Check sheet for the modelled part. Datum: model origin and axes. Units: mm. Face numbers are marked on the shaded views. Give positions to 0.01 mm unless a question says otherwise; leave off trailing zeros. Loops run counter-clockwise (first coordinate to the right, second up) from the corner with the lowest first, then second, coordinate; pieces in that order, holes last. Notation, with made-up numbers: (11.5, 20.5) -> (46.5, 20.5) arc R23 ccw to (46.5, 57.5) -> close; hole circle Ø3 at (27, 9.25). An arc over 180 degrees is marked (long way). Answer as CSV lines item,"result". Start each with the question number.
(1) Gauge pin test, flat ends, axial feed: pin 1 Ø5 at (x, z) = (120, 10.5) entering from -Y; pin 2 Ø0.6 at (y, z) = (3.5, 15.5) entering from -X; pin 3 Ø1.5 at (y, z) = (1.5, 9.5) entering from +X. Record the tip position at first contact, or that the pin passes through.
(2) Release check for a two-part mould opening along Z. For the marked faces 1 and 2 record: pulls with the +Z half, pulls with the -Z half, needs draft (parallel to the pull), parting line crosses it, or undercut.
(3) Section check A-A on x = 51.5. Enter the section's corners in (y, z), plus the area to 3 significant figures.
(4) Material ranges on line 1 (Z direction, x = 3.3, y = 2); line 2 (X direction, y = 0.9, z = 14); line 3 (Y direction, x = 1.4, z = 16), recorded low to high. Write a range as from..to.
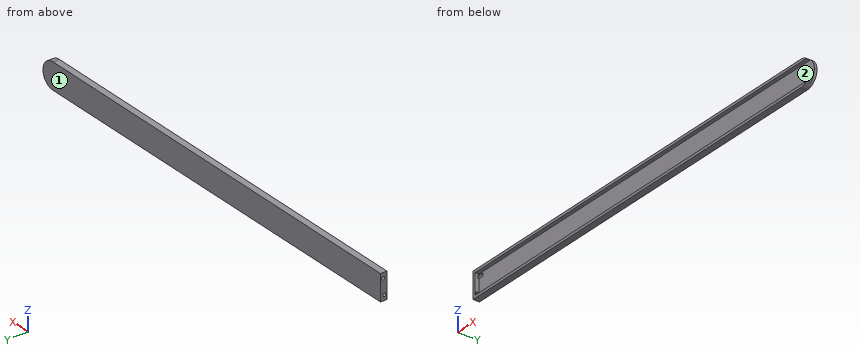
Autodesk Inventor part; units mm, degrees
ref_plane "YZ Plane" through (0, 0, 0) normal (1, 0, 0) x (0, 1, 0)
ref_plane "XZ Plane" through (0, 0, 0) normal (0, 1, 0) x (-1, 0, 0)
ref_plane "XY Plane" through (0, 0, 0) normal (0, 0, 1) x (1, 0, 0)
sketch "スケッチ1" plane through (0, 0, 0) normal (0, 0, 1) x (1, 0, 0)
  line L0 (0, 0) -> (352, 0)
  line L1 (352, 0) -> (352, 5)
  line L2 (352, 5) -> (0, 5)
  line L3 (0, 5) -> (0, 0)
  line L4 (0, 0) -> (6, 0)
  line L5 (0, 1) -> (0, 0)
  dimension "d0" = 352
  dimension "d1" = 5
extrude "押し出し1" add sketch "スケッチ1" along normal blind 20
sketch "スケッチ3" plane through (0, 0, 0) normal (-1, 0, 0) x (0, 0, 1)
  line L0 (0, 5) -> (0, 0)
  line L1 (0, 0) -> (20, 0)
  line L2 (20, 5) -> (20, 0)
  line L3 (0, 5) -> (20, 5)
  circle A0 centre (4, 2) radius 1.2
  circle A1 centre (16, 3) radius 1.2
  dimension "d14" = 2.4
  dimension "d15" = 2.4
  dimension "d16" = 3
  dimension "d17" = 4
  dimension "d18" = 4
  dimension "d19" = 3
extrude "押し出し3" cut sketch "スケッチ3" against normal blind 6 contours A0 | A1
sketch "スケッチ4" plane through (0, 0, 0) normal (0, -1, 0) x (1, 0, 0)
  line L0 (0, 0) -> (352, 0)
  line L1 (352, 0) -> (352, 20)
  line L2 (0, 20) -> (352, 20)
  line L3 (0, 0) -> (0, 20)
  line L4 (2, 2) -> (350, 2)
  line L5 (350, 2) -> (350, 18)
  line L6 (350, 18) -> (2, 18)
  line L7 (2, 18) -> (2, 2)
  dimension "d22" = 2
  dimension "d23" = 2
  dimension "d24" = 2
  dimension "d25" = 2
extrude "押し出し4" cut sketch "スケッチ4" against normal blind 3 contours L7 L6 L5 L4
sketch "スケッチ5" plane through (0, 0, 0) normal (0, 0, -1) x (-1, 0, 0)
  line L0 (-352, 0) -> (-352, 5)
  line L1 (0, 0) -> (-352, 0)
  line L2 (-352, 5) -> (0, 5)
  line L3 (-352, 0) -> (-352, 5)
  line L4 (-352, 5) -> (0, 5)
  line L5 (-352, 0) -> (-340, 0)
  line L6 (-340, 0) -> (-340, 5)
  line L7 (-340, 5) -> (-352, 5)
  line L8 (-352, 5) -> (-352, 0)
  dimension "d28" = 12
extrude "押し出し5" cut sketch "スケッチ5" against normal through all
fillet "フィレット1" radius 10 2 edges at (340, 2.5, 0) (340, 2.5, 20)
properties part number "arm1_L"
Working result:
1,pin 1,"stops at y = 3"
1,pin 2,"stops at x = 6"
1,pin 3,"stops at x = 2"
2,face 1,"needs draft"
2,face 2,"undercut"
3,outline,"(0, 0) -> (5, 0) -> (5, 20) -> (0, 20) -> (0, 18) -> (3, 18) -> (3, 2) -> (0, 2) -> close"
3,area,"52.0 mm^2"
4,line 1,"z = 0..2, 18..20"
4,line 2,"x = 0..2"
4,line 3,"y = 0..1.8, 4.2..5"
